```python
from build123d import *

# Parameters (mm, degrees)
F0_R     = 3.048
F1_DEPTH = 114.3
F3_DEPTH = 25.4
F5_DEPTH = 25.4


with BuildPart() as f1:
    # F0 (on Right) → F1 (new body)
    with BuildSketch(Plane.YZ):
        Circle(F0_R)
    extrude(amount=F1_DEPTH)

    # F2 (on face) → F3 (join)
    with BuildSketch(Plane.YZ.offset(114.3)):
        with BuildLine():
            Line((-12.6839943098, -1.8982821818), (-2.3847072689, -1.8982821818))
            ThreePointArc((-2.3847072689, -1.8982821818), (-3.0479878513, 0.0086057166), (-2.3739500803, 1.9117178182))
            Line((-2.3739500803, 1.9117178182), (-12.6839943098, 1.9117178182))
            Line((-12.6839943098, 1.9117178182), (-12.6839943098, -1.8982821818))
        make_face()
        with BuildLine():
            Line((-2.3847072689, -1.8982821818), (2.3847072689, -1.8982821818))
            ThreePointArc((2.3847072689, -1.8982821818), (2.877402627, -1.0054144032), (3.048, 0))
            ThreePointArc((3.048, 0), (2.8745524734, 1.0135344482), (2.3739500803, 1.9117178182))
            Line((2.3739500803, 1.9117178182), (-2.3739500803, 1.9117178182))
            ThreePointArc((-2.3739500803, 1.9117178182), (-3.0479878513, 0.0086057166), (-2.3847072689, -1.8982821818))
        make_face()
        with BuildLine():
            Line((2.3847072689, -1.8982821818), (12.7160056902, -1.8982821818))
            Line((12.7160056902, -1.8982821818), (12.7160056902, 1.9117178182))
            Line((12.7160056902, 1.9117178182), (2.3739500803, 1.9117178182))
            ThreePointArc((2.3739500803, 1.9117178182), (2.8745524734, 1.0135344482), (3.048, 0))
            ThreePointArc((3.048, 0), (2.877402627, -1.0054144032), (2.3847072689, -1.8982821818))
        make_face()
    extrude(amount=F3_DEPTH)

    # F4 (on face) → F5 (cut)
    with BuildSketch(Plane.XY.offset(1.9117178182)):
        with BuildLine():
            ThreePointArc((114.3, 7.3106571527), (128.51905795, 12.1073757501), (137.3848106384, 0))
            ThreePointArc((137.3848106384, 0), (133.8876655087, -8.751997614), (125.3222181603, -12.6839943098))
            Line((125.3222181603, -12.6839943098), (139.7, -12.6839943098))
            Line((139.7, -12.6839943098), (139.7, 12.7160056902))
            Line((139.7, 12.7160056902), (114.3, 12.7160056902))
            Line((114.3, 12.7160056902), (114.3, 7.3106571527))
        make_face()
        with BuildLine():
            ThreePointArc((124.0474031165, -12.6839943098), (118.5537005151, -11.1220271828), (114.3, -7.3106571527))
            Line((114.3, -7.3106571527), (114.3, -12.6839943098))
            Line((114.3, -12.6839943098), (124.0474031165, -12.6839943098))
        make_face()
    extrude(amount=-F5_DEPTH, mode=Mode.SUBTRACT)


solid = f1.part
```
Source: CAD feature listing. Evaluate the final solid. Frame: model axes, mm. A direction names the side the tool comes from. Coordinates: 2 decimals unless noted, no trailing zeros. Order: outer loops, then holes, each group sorted by start corner. A loop starts at its lowest first (then second) coordinate and runs counter-clockwise, first axis right, second up. Notation, with made-up numbers: M 22.5,73 L 29.5,73 A23 ccw 29.5,86 Z; hole C 46,70.25 d5. An arc over 180 degrees is marked long. Write each question's results on one line, items separated by ' | '. Start each with the question number.
1) Section query B-B (x = 113). Return the cut outline in (y, z).
2) Line query: line 1 (Y direction, x = 41.5, z = 0); line 2 (Z direction, x = 20, y = 0.25); line 3 (Y direction, x = 65, z = 1.25). Output: solid intervals per line, ascending. Write a range as from..to.
3) Section query C-C (y = -8.75). Return the cut outline in (x, z), plus the area to 3 significant figures.
4) Section query A-A (z = 0). Return the cut outline in (x, y), plus the area to 3 significant figures.
5) Contact query for flat-ended pins moving along their axis: pin 1 Ø1.3 at (y, z) = (-1, -2.5) entering from +X; pin 2 Ø0.9 at (y, z) = (-0.5, 2.5) entering from +X; pin 3 Ø2 at (y, z) = (-9, 1.5) entering from +X. Output: stop coordinate, or through.
6) Access query for faces 1 (the face through (56.35, -0.4, 3.02)), 2 (the face through (126, 0, 1.912)), 3 (the face through (126, 0, -1.898)). Directions: +Z, -Z, +X, -X, +Y, -Y. A direction counts if a zero-diameter tool reaches every point of the face in a straight line with its end or side. Return the directions, or none.
Answers:
1) outline: C 0,0 d6.1
2) line 1: y = -3.05..3.05 | line 2: z = -3.04..3.04 | line 3: y = -2.78..2.78
3) outline: M 115.48,-1.9 L 133.89,-1.9 L 133.89,1.91 L 115.48,1.91 Z | area: 70.1 mm^2
4) outline: M 0,-3.05 L 114.3,-3.05 L 114.3,-7.31 A12.7 ccw 124.05,-12.68 L 125.32,-12.68 A12.7 ccw long 114.3,7.31 L 114.3,3.05 L 0,3.05 Z | area: 1,180 mm^2
5) pin 1: stops at x = 137.36 | pin 2: stops at x = 114.3 | pin 3: stops at x = 134.55
6) face 1: -X | face 2: +Z, +X, +Y, -Y | face 3: -Z, +X, +Y, -Y
